```python
from build123d import *

# Parameters (mm, degrees)
CROQUIS2_W              = 26.743660572
CROQUIS2_H              = 8.055392927
CROQUIS2_W_2            = 17.066952721
CROQUIS2_H_2            = 4.555392927
SALIENTE_EXTRUIR1_DEPTH = 5
CORTAR_EXTRUIR1_DEPTH   = 6.055393
SALIENTE_EXTRUIR2_DEPTH = 3.04
CROQUIS7_W              = 10
CROQUIS7_H              = 8.055392927
SALIENTE_EXTRUIR3_DEPTH = 3.04


with BuildPart() as part:
    # Croquis2 → Saliente-Extruir1 (new body, symmetric)
    with BuildSketch(Plane.XY):
        with Locations((11.482548502, 2.027696464)):
            Rectangle(CROQUIS2_W, CROQUIS2_H)
        with Locations((8.53347636, 2.277696464)):
            Rectangle(CROQUIS2_W_2, CROQUIS2_H_2, mode=Mode.SUBTRACT)
    extrude(amount=SALIENTE_EXTRUIR1_DEPTH, both=True)

    # Croquis3 → Cortar-Extruir1 (cut)
    with BuildSketch(Plane(origin=(0, 6.055392927, 0), x_dir=(1, 0, 0), z_dir=(0, 1, 0))):
        Polygon((9, -2.44020423), (9, -1.3), (0, -1.3), (0, 1.3), (9, 1.3), (9, 2.44020423), (18.2, 2.44020423), (18.2, -2.44020423), align=None)
    extrude(amount=-CORTAR_EXTRUIR1_DEPTH, mode=Mode.SUBTRACT)

    # Croquis4 → Saliente-Extruir2 (add)
    with BuildSketch(Plane(origin=(0, 0, 0), x_dir=(1, 0, 0), z_dir=(0, 1, 0))):
        Polygon((17.066952721, 5), (0, 5), (0, -5), (17.066952721, -5), (17.066952721, -2.44020423), (18.2, -2.44020423), (18.2, 2.44020423), (17.066952721, 2.44020423), align=None)
    extrude(amount=SALIENTE_EXTRUIR2_DEPTH)

    # Croquis6 → Revolución1 (revolve)
    with BuildSketch(Plane.XY):
        with BuildLine():
            Line((-1.088241608, 2.027696464), (-16.088241608, 2.027696464))
            ThreePointArc((-16.088241608, 2.027696464), (-8.588241608, 9.527696464), (-1.088241608, 2.027696464))
        make_face()
    revolve(axis=Axis((-1.889281784, 2.027696464, 0), (-1, 0, 0)))

    # Croquis7 → Saliente-Extruir3 (add)
    with BuildSketch(Plane.ZY.offset(1.889281784)):
        with Locations((0, 2.027696464)):
            Rectangle(CROQUIS7_W, CROQUIS7_H)
    extrude(amount=SALIENTE_EXTRUIR3_DEPTH)


solid = part.part
```
Check sheet for the modelled part. Datum: model origin and axes. Units: mm. A direction names the side the tool comes from. Coordinates: 2 decimals unless noted, no trailing zeros. Order: outer loops, then holes, each group sorted by start corner. A loop starts at its lowest first (then second) coordinate and runs counter-clockwise, first axis right, second up. Notation, with made-up numbers: (45, 24.5) -> (102, 24.5) arc R33 ccw to (102, 54.5) -> close; hole circle Ø1 at (-31.5, 63.5). An arc over 180 degrees is marked (long way). Write item = value, one per line. Start each with the question number.
1) Cross-section at D-D (x = 0.5). Enter the section's corners in (y, z), then the cut area to 3 significant figures.
2) Cross-section at C-C (z = 4.25). Enter the section's corners in (x, y).
3) Access from +Z, -Z, +X, -X, +Y, -Y to the whole of each face (thin tool, end or side, straight path). Record for faces 1 (the flat face through (17.067, 4, 4)), 2 (the flat face through (0, 4, 0)), 3 (the flat face through (5, 5, 1.3)).
4) Mould release check, pull along Z, two halves, no side actions. Record for faces 4 (the flat face through (10, 2, -5)), 5 (the flat face through (10, -2, 0)), 6 (the flat face through (18.2, 5, 0)), 7 (the flat face through (4, 5, -1.3)): +Z half, -Z half, draft (parallel to the pull), parting line (faces both ways), or undercut.
5) Material ranges on L1, parallel to Y at x = 11, z = 4.75; L2, parallel to Z at x = 7.5, y = 4.75; L3, parallel to Y at x = -1.5, z = -2.25, recorded low to high.
6) Cross-section at B-B (y = 3.5). Enter the section's corners in (x, z), then the cut area to 3 significant figures.
7) Go/stop test with flat-tipped pins: P1, Ø0.8, axis at y = 4, z = -3, coming from the -X side; P2, Ø2.5, axis at x = 14, y = 1.5, coming from the -Z side; P3, Ø5, axis at x = 6.5, z = 0, coming from the -Y side. Record where each tip stops, or that it passes through.
8) Cross-section at A-A (x = 13.5). Enter the section's corners in (y, z).
Ans:
q1.outline = (-2, -5) -> (3.04, -5) -> (3.04, 5) -> (-2, 5) -> close; (4.56, -5) -> (6.06, -5) -> (6.06, -1.3) -> (4.56, -1.3) -> close; (4.56, 1.3) -> (6.06, 1.3) -> (6.06, 5) -> (4.56, 5) -> close
q1.area = 61.5 mm²
q2.outline = (-3.9, -2) -> (24.85, -2) -> (24.85, 6.06) -> (-3.9, 6.06) arc R6.18 ccw (long way) to start; hole (0, 3.04) -> (17.07, 3.04) -> (17.07, 4.56) -> (0, 4.56) -> close
q3.face_1 = +Z, -Z
q3.face_2 = none
q3.face_3 = +Y
q4.face_4 = -Z half
q4.face_5 = draft
q4.face_6 = undercut
q4.face_7 = undercut
q5.L1 = -2 to 3.04, 4.56 to 6.06
q5.L2 = -5 to -1.3, 1.3 to 5
q5.L3 = -2 to 6.06
q6.outline = (-3.2, -5) -> (0, -5) -> (0, 5) -> (-3.2, 5) arc R7.35 ccw (long way) to start; (17.07, -5) -> (24.85, -5) -> (24.85, 5) -> (17.07, 5) -> (17.07, 2.44) -> (18.2, 2.44) -> (18.2, -2.44) -> (17.07, -2.44) -> close
q6.area = 261 mm²
q7.P1 = -15.38
q7.P2 = -5
q7.P3 = -2
q8.outline = (-2, -5) -> (3.04, -5) -> (3.04, 5) -> (-2, 5) -> close; (4.56, -5) -> (6.06, -5) -> (6.06, -2.44) -> (4.56, -2.44) -> close; (4.56, 2.44) -> (6.06, 2.44) -> (6.06, 5) -> (4.56, 5) -> close
